CAD build for the part. Positions are in the model's coordinates, mm. A direction names the side the tool comes from. Give positions to 0.01 mm unless a question says otherwise; leave off trailing zeros. Loops run counter-clockwise (first coordinate to the right, second up) from the corner with the lowest first, then second, coordinate; pieces in that order, holes last. Notation, with made-up numbers: (-3.5, 47.5) - (33.5, 47.5) arc R14 ccw to (33.5, 66.5) - close; hole circle Ø3 at (-29, 62). An arc over 180 degrees is marked (long way). Return JSON: item names as keys, results as strings.
from build123d import *

# Parameters (mm, degrees)
SKETCH1_W              = 93.16400014
SKETCH1_H              = 13.8938
BACKFACEPATTERN_COUNT  = 6
FRONTFACEPATTERN_COUNT = 4


with BuildPart() as part:
    # Sketch1 → Revolve1 (revolve)
    with BuildSketch(Plane(origin=(0, 0, 0), x_dir=(0, 0, -1), z_dir=(1, 0, 0)), mode=Mode.PRIVATE) as revolve1_sk:
        with Locations((-72.887000006, 29.5656)):
            Rectangle(SKETCH1_W, SKETCH1_H)
    revolve(revolve1_sk.sketch.rotate(Axis((0, 0, 119.469000076), (0, 0, -1)), 90), axis=Axis((0, 0, 119.469000076), (0, 0, -1)))

    # Sketch9 → M6x1.0 Tapped Hole3 (revolve, cut)
    with BuildSketch(Plane(origin=(0, 30.565600032, 26.304999936), x_dir=(0, 1, 0), z_dir=(1, 0, 0))):
        Polygon((0, 0), (0, 16.502151548), (2.5, 15), (2.5, 0), align=None)
    m6x1_0_tapped_hole3 = revolve(axis=Axis((0, 30.565600032, 19.954999936), (0, 0, 1)), mode=Mode.SUBTRACT)

    # BackFacePattern: M6x1.0 Tapped Hole3 ×6 about axis
    backfacepattern_axis = Axis((0, 0, 0), (0, 0, 1))
    for i in range(1, BACKFACEPATTERN_COUNT):
        add(m6x1_0_tapped_hole3.rotate(backfacepattern_axis, i * 360 / BACKFACEPATTERN_COUNT), mode=Mode.SUBTRACT)

    # Sketch6 → M6x1.0 Tapped Hole2 (revolve, cut)
    with BuildSketch(Plane(origin=(0, 31.75, 119.469000076), x_dir=(0, -1, 0), z_dir=(1, 0, 0))):
        Polygon((0, 0), (0, 16.502151548), (2.5, 15), (2.5, 0), align=None)
    m6x1_0_tapped_hole2 = revolve(axis=Axis((0, 31.75, 125.819000076), (0, 0, -1)), mode=Mode.SUBTRACT)

    # FrontFacePattern: M6x1.0 Tapped Hole2 ×4 about axis
    frontfacepattern_axis = Axis((0, 0, 0), (0, 0, 1))
    for i in range(1, FRONTFACEPATTERN_COUNT):
        add(m6x1_0_tapped_hole2.rotate(frontfacepattern_axis, i * 360 / FRONTFACEPATTERN_COUNT), mode=Mode.SUBTRACT)


solid = part.part
1. Which spindle directions (+Z, -Z, +X, -X, +Y, -Y) get a long thin tool onto all of the face, cutting with end or side? Do faces 3 (the face through (-24, -1, 26.305)), 4 (the face through (25.72, -12.9, 33.7)), 5 (the face through (-0.11, 34.248, 112.074)). Say none if no direction does.
Values follow:
{"face 3": "-Z, +X, -X, +Y, -Y", "face 4": "-Z", "face 5": "+Z"}
2. Drill centre lines: probe 1 along Y at (x, z) = (-1, 66); probe 2 along Y at (x, z) = (26, 39); probe 3 along Y at (x, z) = (-7, 47.5). Where is each one in solid material? Low to high.
Values follow:
{"probe 1": "y = -36.5 to -22.6, 22.6 to 36.5", "probe 2": "y = -25.64 to -17.74, -12.83 to 12.83, 17.74 to 25.64", "probe 3": "y = -35.84 to -21.51, 21.51 to 35.84"}
3. Pull direction X, two halves, no side cores. Call faces 1 (the face through (-16, -17, 119.469)), 2 (the face through (34.248, 0.11, 112.074)): +X half, -X half, draft (parallel to the pull), parting line (faces both ways), or undercut.
Values follow:
{"face 1": "draft", "face 2": "undercut"}
4. Cut at A-A, the plane x = -15.5. Write the cut outline in (y, z) (3 decimals).
Values follow:
{"outline": "(-33.059, 26.305) - (-16.473, 26.305) - (-16.473, 119.469) - (-33.059, 119.469) - close; (16.473, 26.305) - (33.059, 26.305) - (33.059, 119.469) - (16.473, 119.469) - close"}
5. Cut at B-B, the plane z = 94. Write the cut outline in (x, y) (1 decimal).
Values follow:
{"outline": "circle Ø73 at (0, 0); hole circle Ø45.2 at (0, 0)"}
6. Drop flat-ended pins along their axis: P1, Ø4, axis at x = -26.47, y = 15.28, coming from the -Z side; P2, Ø4.5, axis at x = 0, y = -30.57, coming from the -Z side; P3, Ø2, axis at x = 17.5, z = 77.5, coming from the -Y side. Give the stop position or say it passes through.
Values follow:
{"P1": "stops at z = 41.6", "P2": "stops at z = 41.45", "P3": "stops at y = -32.57"}
7. Cut at C-C, the plane z = 108. Give the number of separate pieces and of enclosed holes in the cut face, plus the area to 3 significant figures.
Values follow:
{"separate pieces": "1", "enclosed holes": "5", "area": "2,500 mm²"}
